Build history of the part. All positions in model axes, mm. Face numbers are marked on the shaded views. A direction names the side the tool comes from. Coordinates: 2 decimals unless noted, no trailing zeros. Loops run counter-clockwise (first coordinate to the right, second up) from the corner with the lowest first, then second, coordinate; pieces in that order, holes last. Notation, with made-up numbers: M 67.5,37 L 124.5,37 A21 cw 124.5,60 Z; hole C 77,24.25 d1. An arc over 180 degrees is marked long. Write each question's results on one line, items separated by ' | '. Start each with the question number.
from build123d import *

# Parameters (mm, degrees)
SKETCH1_W           = 19.05
SKETCH1_H           = 19.05
BOSS_EXTRUDE1_DEPTH = 19.05
SKETCH2_W           = 15.875
SKETCH2_H           = 15.875
BOSS_EXTRUDE2_DEPTH = 28.575
SKETCH3_W           = 15.875
SKETCH3_H           = 15.875
BOSS_EXTRUDE3_DEPTH = 28.575
SKETCH4_W           = 15.875
SKETCH4_H           = 15.875
BOSS_EXTRUDE4_DEPTH = 28.575


with BuildPart() as part:
    # Sketch1 → Boss-Extrude1 (new body)
    with BuildSketch(Plane.XY):
        Rectangle(SKETCH1_W, SKETCH1_H)
    extrude(amount=BOSS_EXTRUDE1_DEPTH)

    # Sketch2 → Boss-Extrude2 (add)
    with BuildSketch(Plane(origin=(0, 9.525, 0), x_dir=(1, 0, 0), z_dir=(0, 1, 0))):
        with Locations((0, -9.525)):
            Rectangle(SKETCH2_W, SKETCH2_H)
    extrude(amount=BOSS_EXTRUDE2_DEPTH)

    # Sketch3 → Boss-Extrude3 (add)
    with BuildSketch(Plane(origin=(9.525, 0, 0), x_dir=(0, 0, -1), z_dir=(1, 0, 0))):
        with Locations((-9.525, 0)):
            Rectangle(SKETCH3_W, SKETCH3_H)
    extrude(amount=BOSS_EXTRUDE3_DEPTH)

    # Sketch4 → Boss-Extrude4 (add)
    with BuildSketch(Plane.XY.offset(19.05)):
        Rectangle(SKETCH4_W, SKETCH4_H)
    extrude(amount=BOSS_EXTRUDE4_DEPTH)


solid = part.part
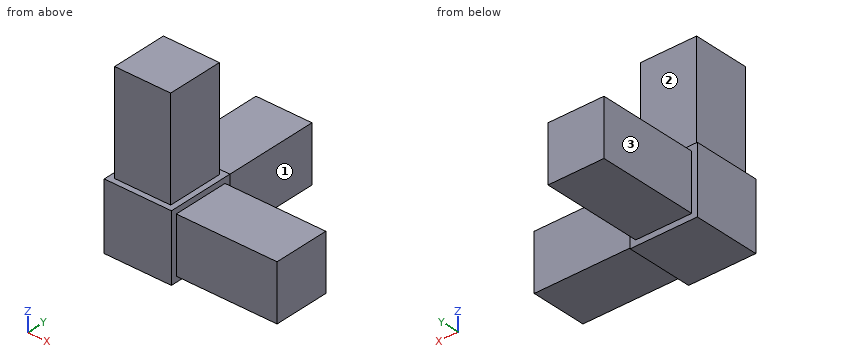
1. Band-saw the part on A-A, the plane z = 14.5. List the corners of the cut face in (x, y) (1 decimal).
2. Wall check: line 1 along X through (y, z) = (32, 8); line 2 along Z through (x, y) = (-5, 23). Give the ranges that are in metal, low to high.
3. Pin check, flat tips, straight feed: pin 1 (5 mm diameter, centred on x = 1.5, z = 27, fed in from -Y); pin 2 (2 mm diameter, centred on y = 7.5, z = 37.5, fed in from -X); pin 3 (8 mm diameter, centred on y = 29.5, z = 6.5, fed in from +X). Stop position of each tip, or through.
4. Band-saw the part on D-D, the plane z = 31. List the corners of the cut face in (x, y).
5. Which spindle directions (+Z, -Z, +X, -X, +Y, -Y) get a long thin tool onto all of the face, cutting with end or side? Do the marked faces 1, 2 and 3. Say none if no direction does.
6. Band-saw the part on C-C, the plane y = 30.5. List the corners of the cut face in (x, z).
Checked values:
1) outline: M -9.5,-9.5 L 9.5,-9.5 L 9.5,-7.9 L 38.1,-7.9 L 38.1,7.9 L 9.5,7.9 L 9.5,9.5 L 7.9,9.5 L 7.9,38.1 L -7.9,38.1 L -7.9,9.5 L -9.5,9.5 Z
2) line 1: -7.94 to 7.94 | line 2: 1.59 to 17.46
3) pin 1: y = -7.94 | pin 2: x = -7.94 | pin 3: x = 7.94
4) outline: M -7.94,-7.94 L 7.94,-7.94 L 7.94,7.94 L -7.94,7.94 Z
5) face 1: +Z, -Z, +X, +Y | face 2: +Z, +X, -X, +Y | face 3: +Z, -Z, -X, +Y
6) outline: M -7.94,1.59 L 7.94,1.59 L 7.94,17.46 L -7.94,17.46 Z
